from build123d import *

# Parameters (mm, degrees)
F0_W     = 21.1
F0_H     = 15.8
F1_DEPTH = 1.6
F2_R     = 1.625
F3_DEPTH = 25
F4_W     = 4
F4_H     = 4
F5_DEPTH = 1.5
F6_R     = 0.5
F7_DEPTH = 25


with BuildPart() as f1:
    # F0 (on Top) → F1 (new body)
    with BuildSketch(Plane.XY):
        Rectangle(F0_W, F0_H)
    extrude(amount=F1_DEPTH)

    # F2 (on face) → F3 (cut)
    with BuildSketch(Plane.XY.offset(1.6)):
        with Locations((8.3, 5.65)):
            Circle(F2_R)
        with Locations((8.3, -5.65)):
            Circle(F2_R)
    extrude(amount=-F3_DEPTH, mode=Mode.SUBTRACT)

    # F4 (on face) → F5 (join)
    with BuildSketch(Plane.XY.offset(1.6)):
        Rectangle(F4_W, F4_H)
    extrude(amount=F5_DEPTH)

    # F6 (on face) → F7 (cut)
    with BuildSketch(Plane.XY.offset(1.6)):
        with Locations((-8.989307, 4.4)):
            Circle(F6_R)
        with Locations((-8.989307, 2.4)):
            Circle(F6_R)
        with Locations((-8.989307, 0.4)):
            Circle(F6_R)
        with Locations((-8.989307, -1.6)):
            Circle(F6_R)
        with Locations((-8.989307, -3.6)):
            Circle(F6_R)
    extrude(amount=-F7_DEPTH, mode=Mode.SUBTRACT)


solid = f1.part
The model under review builds one solid part; all positions refer to its coordinate system, in mm. A direction names the side the tool comes from. Give positions to 0.01 mm unless a question says otherwise; leave off trailing zeros. Order: outer loops, then holes, each group sorted by start corner. A loop starts at its lowest first (then second) coordinate and runs counter-clockwise, first axis right, second up. Notation, with made-up numbers: M 58.25,-38 L 68.25,-38 A18 cw 68.25,-11 Z; hole C -29,62.25 d11. An arc over 180 degrees is marked long. Use one line per item in the form item = value. Start each with the question number.
Item 1: For faces 4 (the flat face through (10.55, 0, 1)), 5 (the flat face through (2, 0, 2)), 6 (the flat face through (-2, 0, 2)), 7 (the flat face through (0, -2, 2)), 8 (the flat face through (0, 0, 3.1)), list the 3-axis set-ups (+Z, -Z, +X, -X, +Y, -Y) from which the entire face can be reached by the end or side of a thin tool; tool diameter is ignored.
Item 2: We need section C-C on y = 0.4. Give the boundary of the cut face in (x, z), plus the area to 3 significant figures.
Item 3: We need section A-A on z = 0.3. Give the boundary of the cut face in (x, y) (3 decimals).
Item 4: The part is to be moulded in two halves that separate along Y. For faces 1 (the flat face through (0, 2, 2)), 2 (the flat face through (-2.5, 0.1, 1.6)), 3 (the cylindrical face through (-8.512, 0.55, 0.811)), say which applies: pulls with the +Y half, pulls with the -Y half, needs draft (parallel to the pull), parting line crosses it, or undercut.
Item 5: We need section D-D on y = 4.4. Give the boundary of the cut face in (x, z).
Item 6: To check wall thickness, follow line 1 along Y through (x, z) = (8.3, 1.1) (3 decimals); line 2 along Z through (x, y) = (6, -7); line 3 along X through (y, z) = (-4.75, 0.85). State the ranges of each line that lie inside material, in increasing order. Write a range as from..to.
Item 7: Insertion check: pin 1 Ø4 at (x, y) = (5.5, 4.5) entering from -Z; pin 2 Ø0.8 at (x, z) = (-1, 2.5) entering from +Y; pin 3 Ø4 at (x, y) = (4, 4) entering from +Z. Each pin has a flat end and moves straight along its axis. Give the tip position at first contact, or say it passes through.
Item 8: We need section B-B on x = 8.3. Give the boundary of the cut face in (y, z) (3 decimals).
Completed:
q1.face_4 = +Z, -Z, +X, +Y, -Y
q1.face_5 = +Z, +X, +Y, -Y
q1.face_6 = +Z, -X, +Y, -Y
q1.face_7 = +Z, +X, -X, -Y
q1.face_8 = +Z, +X, -X, +Y, -Y
q2.outline = M -10.55,0 L -9.49,0 L -9.49,1.6 L -10.55,1.6 Z; M -8.49,0 L 10.55,0 L 10.55,1.6 L 2,1.6 L 2,3.1 L -2,3.1 L -2,1.6 L -8.49,1.6 Z
q2.area = 38.2 mm²
q3.outline = M -10.55,-7.9 L 10.55,-7.9 L 10.55,7.9 L -10.55,7.9 Z; hole C -8.989,-3.6 d1; hole C -8.989,-1.6 d1; hole C -8.989,0.4 d1; hole C -8.989,2.4 d1; hole C -8.989,4.4 d1; hole C 8.3,-5.65 d3.25; hole C 8.3,5.65 d3.25
q4.face_1 = pulls with the +Y half
q4.face_2 = needs draft
q4.face_3 = undercut
q5.outline = M -10.55,0 L -9.49,0 L -9.49,1.6 L -10.55,1.6 Z; M -8.49,0 L 7.26,0 L 7.26,1.6 L -8.49,1.6 Z; M 9.34,0 L 10.55,0 L 10.55,1.6 L 9.34,1.6 Z
q6.line_1 = -7.9..-7.275, -4.025..4.025, 7.275..7.9
q6.line_2 = 0..1.6
q6.line_3 = -10.55..6.95, 9.65..10.55
q7.pin_1 = 0
q7.pin_2 = 2
q7.pin_3 = 1.6
q8.outline = M -7.9,0 L -7.275,0 L -7.275,1.6 L -7.9,1.6 Z; M -4.025,0 L 4.025,0 L 4.025,1.6 L -4.025,1.6 Z; M 7.275,0 L 7.9,0 L 7.9,1.6 L 7.275,1.6 Z
